Read the model definition and answer for the solid it produces. Units are mm, in the model's axes. Round coordinates to 2 decimals unless told otherwise and drop trailing zeros. Order: outer loops, then holes, each group sorted by start corner. A loop starts at its lowest first (then second) coordinate and runs counter-clockwise, first axis right, second up. Notation, with made-up numbers: (64, 63) - (71, 63) arc R28 cw to (71, 102) - close; hole circle Ø6 at (45.25, 6.5). An arc over 180 degrees is marked (long way). Put each result on its own line as item: value. Start each with the question number.
Q1. Section C-C on y = 1.75 is taken. State how many separate pieces and enclosed holes the cut face has, then the cut area to 3 significant figures.
Q2. For a pull along X with two mould halves and no side action, classify faces 1 (the face through (75.537, 5.07, 15.298)), 2 (the face through (77.49, 5.07, 57.15)), 3 (the face through (-1, 5, -60)), 4 (the face through (-77.65, 5.07, -56.99)) as pulls with the +X half, pulls with the -X half, needs draft (parallel to the pull), parting line crosses it, or undercut.
Q3. Section A-A on x = -65.5 is taken. Give the vertices of the cut face in (y, z), then the cut area to 3 significant figures.
Q4. Find the intervals of material crossed by line 1 along X through (y, z) = (6.25, -1); line 2 along X through (y, z) = (3.5, 45); line 3 along X through (y, z) = (5, -8), in increasing order. Write a range as from..to.
Q5. Section B-B on z = -45 is taken. Give the vertices of the cut face in (x, y).
Q6. This flat-tipped pin is pushed along its axis until it touches: pin 1 Ø6 at (x, z) = (-20.5, -45) entering from +Y. Where does it stop, or does it pass through?
from build123d import *

# Parameters (mm, degrees)
SKETCH_1_W          = 161
SKETCH_1_H          = 120
EXTRUDE_1_DEPTH     = 10
FILLET_1_R          = 10
SKETCH_2_R          = 1.55
CUT_EXTRUDE_1_DEPTH = 10
SKETCH_3_R          = 16.5
CUT_EXTRUDE_2_DEPTH = 10
SKETCH_4_R          = 3.4
CUT_EXTRUDE_3_DEPTH = 101.897224937


with BuildPart() as part:
    # 草图1 → 凸台-拉伸1 (new body)
    with BuildSketch(Plane(origin=(0, 0, 0), x_dir=(1, 0, 0), z_dir=(0, 1, 0))):
        Rectangle(SKETCH_1_W, SKETCH_1_H)
    extrude(amount=EXTRUDE_1_DEPTH)

    # 圆角1
    fillet_1_edges = [part.edges().sort_by_distance(p)[0] for p in [
        (80.5, 5, 60),
        (-80.5, 5, 60),
        (-80.5, 5, -60),
        (80.5, 5, -60),
    ]]
    fillet(fillet_1_edges, radius=FILLET_1_R)

    # 草图2 → 切除-拉伸1 (cut)
    with BuildSketch(Plane(origin=(0, 10, 0), x_dir=(1, 0, 0), z_dir=(0, 1, 0))):
        with Locations(Location((74, 15.5, 0), (0, 0, 270))):
            Circle(SKETCH_2_R)
        with Locations(Location((74, -15.5, 0), (0, 0, 270))):
            Circle(SKETCH_2_R)
        with Locations(Location((43, 15.5, 0), (0, 0, 270))):
            Circle(SKETCH_2_R)
        with Locations(Location((43, -15.5, 0), (0, 0, 270))):
            Circle(SKETCH_2_R)
    extrude(amount=-CUT_EXTRUDE_1_DEPTH, mode=Mode.SUBTRACT)

    # 草图3 → 切除-拉伸2 (cut)
    with BuildSketch(Plane.XZ):
        with Locations(Location((58.5, 0, 0), (0, 0, 270))):
            Circle(SKETCH_3_R)
    extrude(amount=-CUT_EXTRUDE_2_DEPTH, mode=Mode.SUBTRACT)

    # 草图4 → 切除-拉伸3 (cut, through all)
    with BuildSketch(Plane.XZ):
        with Locations(Location((-20.5, 45, 0), (0, 0, 270))):
            Circle(SKETCH_4_R)
        with Locations(Location((-65.5, 0, 0), (0, 0, 270))):
            Circle(SKETCH_4_R)
        with Locations(Location((-20.5, -45, 0), (0, 0, 270))):
            Circle(SKETCH_4_R)
    extrude(amount=-CUT_EXTRUDE_3_DEPTH, mode=Mode.SUBTRACT)


solid = part.part
Findings:
1. separate pieces: 1
1. enclosed holes: 8
1. area: 18,200 mm2
2. face 1: undercut
2. face 2: pulls with the +X half
2. face 3: needs draft
2. face 4: pulls with the -X half
3. outline: (0, -60) - (10, -60) - (10, -3.4) - (0, -3.4) - close; (0, 3.4) - (10, 3.4) - (10, 60) - (0, 60) - close
3. area: 1,130 mm2
4. line 1: -80.5..-68.75, -62.25..42.03, 74.97..80.5
4. line 2: -80.5..-23.9, -17.1..80.5
4. line 3: -80.5..44.07, 72.93..80.5
5. outline: (-80.5, 0) - (-23.9, 0) - (-23.9, 10) - (-80.5, 10) - close; (-17.1, 0) - (80.5, 0) - (80.5, 10) - (-17.1, 10) - close
6. pin 1: through
